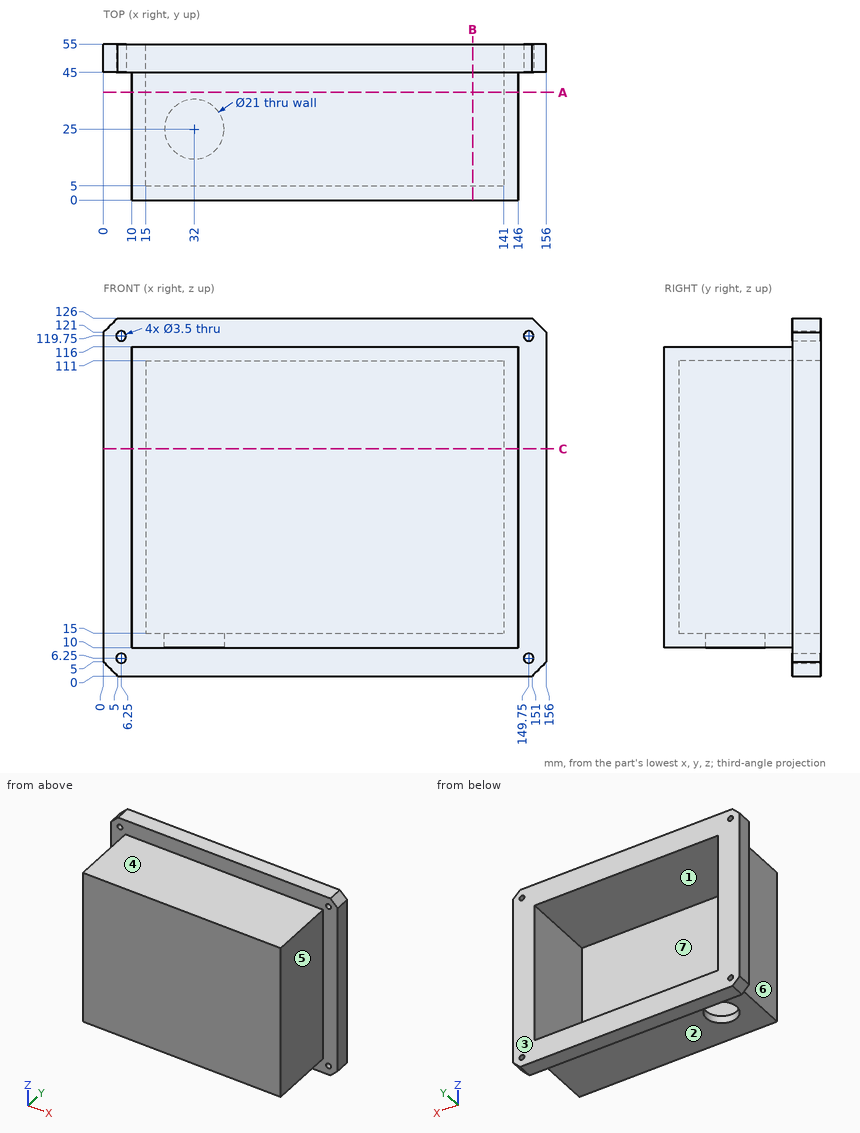
Design review of the part shown in the three views and the two pictorial views. Dimensions are in mm from the part's minimum x, y and z. A direction names the side the tool comes from. Round coordinates to 2 decimals unless told otherwise and drop trailing zeros. Order: outer loops, then holes, each group sorted by start corner. A loop starts at its lowest first (then second) coordinate and runs counter-clockwise, first axis right, second up.
Q1. Machinability: for the marked faces 5, 6 and 7, which of the approach directions +Z, -Z, +X, -X, +Y, -Y give a long, thin tool a straight path to every point of the face, cutting with its end or side? Answer none if there is none.
Findings below:
face 5: +Z, -Z, +X, -Y
face 6: +Z, -Z, -X, -Y
face 7: +Y
Q2. Insertion check: P1, Ø8, axis at y = 24, z = 95, coming from the +X side; P2, Ø4, axis at x = 77.5, y = 9, coming from the +Z side; P3, Ø5.5, axis at x = 149.75, z = 119.75, coming from the -Y side; P4, Ø2, axis at x = 6.25, z = 6.25, coming from the +Y side. Each pin has a flat end and moves straight along its axis. Give the tip position at first contact, or say it passes through.
Findings below:
P1: stops at x = 146
P2: stops at z = 116
P3: stops at y = 45
P4: passes through
Q3. We need section C-C, the plane z = 80. Give the boundary of the cut face in (x, y).
Findings below:
outline: (0, 45) - (10, 45) - (10, 0) - (146, 0) - (146, 45) - (156, 45) - (156, 55) - (141, 55) - (141, 5) - (15, 5) - (15, 55) - (0, 55) - close
Q4. We need section A-A, the plane y = 38. Give the boundary of the cut face in (x, z).
Findings below:
outline: (10, 10) - (146, 10) - (146, 116) - (10, 116) - close; hole (15, 15) - (141, 15) - (141, 111) - (15, 111) - close
Q5. Mouldability with a two-part tool opening along Z and no side actions: class the marked faces 1, 2, 3 and 4 as pulls with the +Z half, pulls with the -Z half, needs draft (parallel to the pull), parting line crosses it, or undercut.
Findings below:
face 1: undercut
face 2: pulls with the -Z half
face 3: needs draft
face 4: pulls with the +Z half
Q6. We need section B-B, the plane x = 130. Give the boundary of the cut face in (y, z).
Findings below:
outline: (0, 10) - (45, 10) - (45, 0) - (55, 0) - (55, 15) - (5, 15) - (5, 111) - (55, 111) - (55, 126) - (45, 126) - (45, 116) - (0, 116) - close
Q7. Wall thickness on line 1 (X direction, y = 51, z = 6); line 2 (Z direction, x = 149.75, y = 49.5); line 3 (X direction, y = 20, z = 69): over which ranges is each line inside the solid? List them lowest first.
Findings below:
line 1: x = 0 to 4.52, 7.98 to 148.02, 151.48 to 156
line 2: z = 0 to 4.5, 8 to 118, 121.5 to 126
line 3: x = 10 to 15, 141 to 146
